Part model, mm, in its own coordinate system. Give positions to 0.01 mm unless a question says otherwise; leave off trailing zeros. Write each loop counter-clockwise with the first axis right and the second up, starting at its lowest first coordinate (ties: lowest second). Pieces come first, ordered by that corner, then holes. Notation, with made-up numbers: (3, -11.5) - (43, -11.5) arc R12 cw to (43, -0.5) - close; hole circle Ø7 at (-36, -24). An arc over 180 degrees is marked (long way). Answer as a JSON object with one key per item and string values. Group by question number.
Autodesk Inventor part; units mm, degrees
ref_plane "YZ Plane" through (0, 0, 0) normal (1, 0, 0) x (0, 1, 0)
ref_plane "XZ Plane" through (0, 0, 0) normal (0, 1, 0) x (-1, 0, 0)
ref_plane "XY Plane" through (0, 0, 0) normal (0, 0, 1) x (1, 0, 0)
sketch "Sketch1" plane through (0, 0, 0) normal (0, 0, 1) x (1, 0, 0)
  circle A0 centre (0, 0) radius 2.3813
  line L0 (0, 0) -> (-19.05, 0) construction
  line L1 (0, 4.7625) -> (-19.05, 4.7625)
  line L2 (-19.05, -4.7625) -> (0, -4.7625)
  arc A1 (0, -4.7625) -> (0, 4.7625) centre (0, 0) ccw
  arc A2 (-19.05, 4.7625) -> (-19.05, -4.7625) centre (-19.05, 0) ccw
  point P0 (-9.525, 0)
  dimension "d0" = 4.7625
  dimension "d2" = 19.05
  dimension "d3" = 9.525
extrude "Extrusion1" add sketch "Sketch1" along normal blind 4.7625
fillet "Fillet1" radius 1.5875 4 edges at (4.7625, 0, 4.7625) (-9.525, 4.7625, 4.7625) (-23.8125, 0, 4.7625) (-9.525, -4.7625, 4.7625)
properties part number "Stands"
1) Probe line 1 (Y direction, x = 0, z = 1.05); line 2 (X direction, y = 1.75, z = 3.65); line 3 (X direction, y = 1, z = 4.5). List the from-to ranges inside material, lowest first.
2) Band-saw the part on B-B (y = 0). List the corners of the cut face in (x, z) (1 decimal).
3) Drop flat-ended pins along their axis: P1, Ø1.5, axis at x = 1, z = 1.5, coming from the +Y side; P2, Ø1.5, axis at y = 3.5, z = 0.5, coming from the -X side. Give the stop position or say it passes through.
4) Band-saw the part on A-A (x = -1.5). List the corners of the cut face in (y, z) (1 decimal).
5) Band-saw the part on D-D (x = -9.75). List the corners of the cut face in (y, z) (1 decimal), plus the area to 3 significant figures.
6) Mould opens along X. For faces 1 (the cylindrical face through (-9.392, -4.285, 4.31)), 2 (the cylindrical face through (-23.81, -0.1, 1.57)), 3 (the cylindrical face through (1.1, 2.11, 2.35)) say: pulls with the +X half, pulls with the -X half, needs draft (parallel to the pull), parting line crosses it, or undercut.
Verdict:
{
 "1": {"line 1": "-4.76 to -2.38, 2.38 to 4.76", "line 2": "-23.4 to -1.61, 1.61 to 4.35", "line 3": "-22.97 to -2.16, 2.16 to 3.92"},
 "2": {"outline": "(-23.8, 0) - (-2.4, 0) - (-2.4, 4.8) - (-22.2, 4.8) arc R1.6 ccw to (-23.8, 3.2) - close; (2.4, 0) - (4.8, 0) - (4.8, 3.2) arc R1.6 ccw to (3.2, 4.8) - (2.4, 4.8) - close"},
 "3": {"P1": "y = 4.76", "P2": "x = -22.94"},
 "4": {"outline": "(-4.8, 0) - (-1.8, 0) - (-1.8, 4.8) - (-3.2, 4.8) arc R1.6 ccw to (-4.8, 3.2) - close; (1.8, 0) - (4.8, 0) - (4.8, 3.2) arc R1.6 ccw to (3.2, 4.8) - (1.8, 4.8) - close"},
 "5": {"outline": "(-4.8, 0) - (4.8, 0) - (4.8, 3.2) arc R1.6 ccw to (3.2, 4.8) - (-3.2, 4.8) arc R1.6 ccw to (-4.8, 3.2) - close", "area": "44.3 mm2"},
 "6": {"face 1": "needs draft", "face 2": "pulls with the -X half", "face 3": "undercut"}
}
